Answer from the drawing. Dimensions are ordinates in mm from the lowest x, y and z of the part. Give positions to 0.01 mm unless a question says otherwise; leave off trailing zeros. Write each loop counter-clockwise with the first axis right and the second up, starting at its lowest first coordinate (ties: lowest second). Pieces come first, ordered by that corner, then holes. Notation, with made-up numbers: (-6.5, 89.25) -> (0.5, 89.25) arc R29 cw to (0.5, 117.25) -> close; hole circle Ø5 at (59.25, 31). An arc over 180 degrees is marked (long way). Write item = value, one per line.
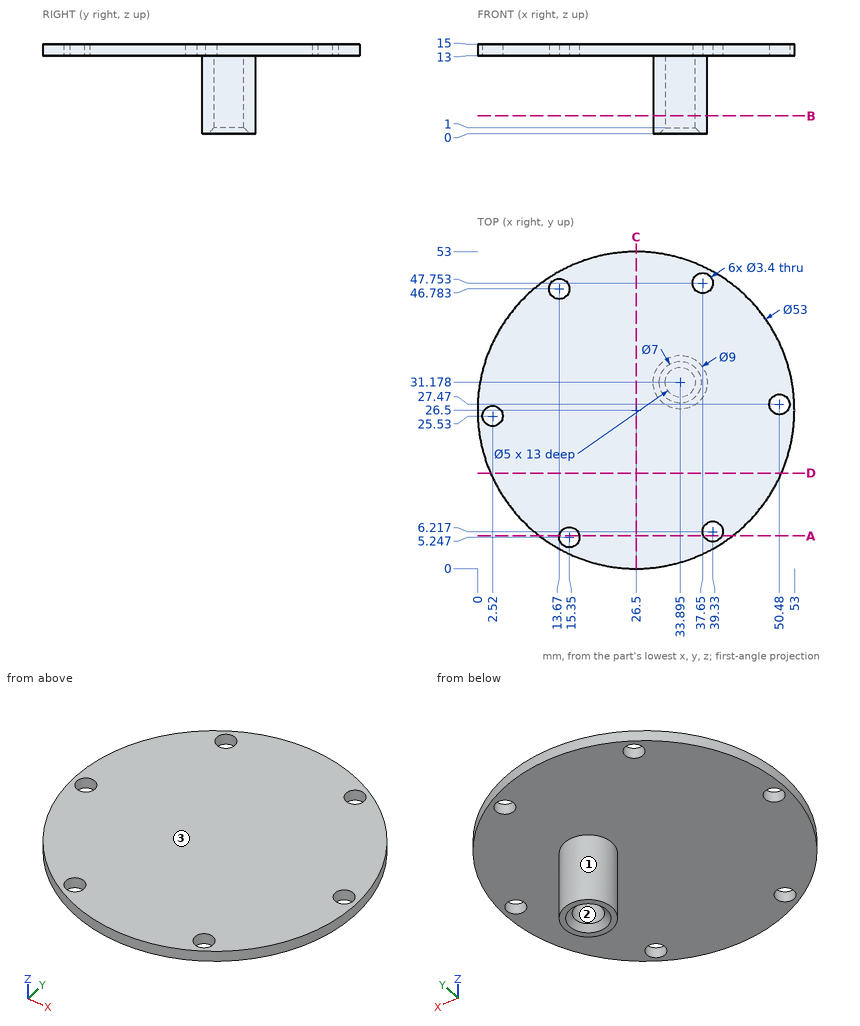
(1) The part is cut by section A-A on y = 5.5. Determine the outline of the cut face in (x, z).
Checks:
outline = (10.34, 13) -> (13.67, 13) -> (13.67, 15) -> (10.34, 15) -> close; (17.03, 13) -> (37.79, 13) -> (37.79, 15) -> (17.03, 15) -> close; (40.87, 13) -> (42.66, 13) -> (42.66, 15) -> (40.87, 15) -> close
(2) The part is cut by section D-D on y = 16. Determine the outline of the cut face in (x, z).
Checks:
outline = (2.17, 13) -> (50.83, 13) -> (50.83, 15) -> (2.17, 15) -> close
(3) For a pull along Y with two mould halves and no side action, classify the marked faces 1, 2 and 3 as released by +Y, released by -Y, zero draft, split by the parting line, or undercut.
Checks:
face_1 = split by the parting line
face_2 = undercut
face_3 = zero draft
(4) Given P1, Ø1.5, axis at y = 42, z = 10.5, coming from the -X side; P2, Ø5.5, axis at x = 39.33, y = 6.22, coming from the +Z side; P3, Ø2, axis at x = 15, y = 23.5, coming from the -Z side; P4, Ø3, axis at x = 36, z = 5, coming from the +Y side, each flat-ended and moving along its own axis, determine where each tip first touches the part or whether it passes through.
Checks:
P1 = through
P2 = 15
P3 = 13
P4 = 35.64
(5) The part is cut by section B-B on z = 3. Determine the outline of the cut face in (x, y) (1 decimal).
Checks:
outline = circle Ø9 at (33.9, 31.2); hole circle Ø5 at (33.9, 31.2)
(6) The part is cut by section C-C on x = 26.5. Determine the outline of the cut face in (y, z), plus the area to 3 significant figures.
Checks:
outline = (0, 13) -> (53, 13) -> (53, 15) -> (0, 15) -> close
area = 106 mm²
(7) Consider L1, parallel to Y at x = 34, z = 8 (1 decimal); L2, parallel to Z at x = 23.5, y = 10; L3, parallel to Y at x = 33.5, z = 7.75 (1 decimal). Determine where each line is inside the solid, lowest interval first.
Checks:
L1 = 26.7 to 28.7, 33.7 to 35.7
L2 = 13 to 15
L3 = 26.7 to 28.7, 33.6 to 35.7
